Work out the finished part from the listing and answer in its coordinate system (mm). A direction names the side the tool comes from. Give positions to 0.01 mm unless a question says otherwise; leave off trailing zeros. Order: outer loops, then holes, each group sorted by start corner. A loop starts at its lowest first (then second) coordinate and runs counter-clockwise, first axis right, second up. Notation, with made-up numbers: (28.25, -23.5) - (33.25, -23.5) arc R28 ccw to (33.25, 14.5) - close; hole circle Ø6 at (68.25, 11.25). An arc over 180 degrees is marked (long way). Write each question's results on one line, items separated by ' | '.
from build123d import *
from build123d.topology import SkipClean

# Parameters (mm, degrees)
SKETCH1_W           = 18
SKETCH1_H           = 20
BOSS_EXTRUDE1_DEPTH = 18
SKETCH6_R           = 7.25
BOSS_EXTRUDE4_DEPTH = 12
FILLET1_R           = 2
SKETCH2_R           = 6.575
SKETCH2_R_2         = 5.625
BOSS_EXTRUDE5_DEPTH = 10
BOSS_EXTRUDE6_START = 10
SKETCH3_R           = 6.575
SKETCH3_R_2         = 5.625
BOSS_EXTRUDE6_DEPTH = 10
SKETCH7_R           = 5.625
CUT_EXTRUDE2_DEPTH  = 41
SKETCH8_W           = 18
SKETCH8_H           = 20
BOSS_EXTRUDE7_DEPTH = 3


with BuildPart() as part:
    # Sketch1 → Boss-Extrude1 (new body)
    with BuildSketch(Plane(origin=(0, 0, 0), x_dir=(1, 0, 0), z_dir=(0, 1, 0))):
        Rectangle(SKETCH1_W, SKETCH1_H)
    extrude(amount=BOSS_EXTRUDE1_DEPTH)

    # Sketch6 → Boss-Extrude4 (add)
    with BuildSketch(Plane(origin=(0, 18, 0), x_dir=(1, 0, 0), z_dir=(0, 1, 0))):
        with Locations(Location((0, 0, 0), (0, 0, 270))):
            Circle(SKETCH6_R)
    extrude(amount=BOSS_EXTRUDE4_DEPTH)

    # Fillet1
    fillet1_edges = [part.edges().sort_by_distance(p)[0] for p in [
        (0, 18, -7.25),
        (0, 30, -7.25),
    ]]
    fillet(fillet1_edges, radius=FILLET1_R)

    # Sketch2 → Boss-Extrude5 (add)
    with BuildSketch(Plane.XY.offset(10)):
        with Locations(Location((0, 9, 0), (0, 0, 180))):
            Circle(SKETCH2_R)
        with Locations((0, 9)):
            Circle(SKETCH2_R_2, mode=Mode.SUBTRACT)
    extrude(amount=BOSS_EXTRUDE5_DEPTH)

    # Sketch3 → Boss-Extrude6 (add)
    with BuildSketch(Plane(origin=(0, 0, -10), x_dir=(-1, 0, 0), z_dir=(0, 0, -1)).offset(BOSS_EXTRUDE6_START)):
        with Locations((0, 9)):
            Circle(SKETCH3_R)
        with Locations(Location((0, 9, 0), (0, 0, 180))):
            Circle(SKETCH3_R_2, mode=Mode.SUBTRACT)
    extrude(amount=-BOSS_EXTRUDE6_DEPTH)

    # Sketch7 → Cut-Extrude2 (cut)
    with SkipClean():  # the faces are left unmerged after this step: merging them gives an invalid solid
        with BuildSketch(Plane(origin=(0, 0, -10), x_dir=(-1, 0, 0), z_dir=(0, 0, -1))):
            with Locations((0, 9)):
                Circle(SKETCH7_R)
        extrude(amount=-CUT_EXTRUDE2_DEPTH, mode=Mode.SUBTRACT)

    # Sketch8 → Boss-Extrude7 (add)
    with SkipClean():  # the faces are left unmerged after this step: merging them gives an invalid solid
        with BuildSketch(Plane.XZ):
            Rectangle(SKETCH8_W, SKETCH8_H)
        extrude(amount=BOSS_EXTRUDE7_DEPTH)


solid = part.part
1. A cutting plane is placed at B-B, the plane y = 14. Write down the section's boundary in (x, z), then the cut area to 3 significant figures.
Answer list:
outline: (-9, -10) - (-4.27, -10) - (-4.27, -20) - (-2.58, -20) - (-2.58, 20) - (-4.27, 20) - (-4.27, 10) - (-9, 10) - close; (2.58, -20) - (4.27, -20) - (4.27, -10) - (9, -10) - (9, 10) - (4.27, 10) - (4.27, 20) - (2.58, 20) - close | area: 325 mm^2
2. A cutting plane is placed at A-A, the plane x = 0. Write down the section's boundary in (y, z) (3 decimals).
Answer list:
outline: (-3, -10) - (2.425, -10) - (2.425, -20) - (3.375, -20) - (3.375, 20) - (2.425, 20) - (2.425, 10) - (-3, 10) - close; (14.625, -20) - (15.575, -20) - (15.575, -10) - (18, -10) - (18, -9.25) arc R2 cw to (20, -7.25) - (28, -7.25) arc R2 ccw to (30, -5.25) - (30, 5.25) arc R2 ccw to (28, 7.25) - (20, 7.25) arc R2 cw to (18, 9.25) - (18, 10) - (15.575, 10) - (15.575, 20) - (14.625, 20) - close
3. Straight lines are drawn through the part: line 1 (X direction, y = 9, z = -5.5) (3 decimals); line 2 (Y direction, x = 0, z = 4.5) (3 decimals); line 3 (Y direction, x = 0, z = -12.5) (3 decimals). For each, find the intervals that lie inside material, in ascending order. Write a range as [from, to].
Answer list:
line 1: [-9, -5.625], [5.625, 9] | line 2: [-3, 3.375], [14.625, 30] | line 3: [2.425, 3.375], [14.625, 15.575]
4. Given P1, Ø8, axis at x = -1.5, y = 23.5, coming from the +Z side; P2, Ø9, axis at x = 0, y = 9, coming from the -Z side; P3, Ø3, axis at x = 1.5, y = 26.5, coming from the -Z side, each flat-ended and moving along its own axis, determine where each tip first touches the part or whether it passes through.
Answer list:
P1: z = 7.27 | P2: through | P3: z = -7.25
5. A cutting plane is placed at C-C, the plane z = -15.5. Write down the section's boundary in (x, y) (3 decimals).
Answer list:
outline: circle Ø13.15 at (0, 9); hole circle Ø11.25 at (0, 9)
6. A tool of negligible diameter and unlimited length cuts with its end or side. For faces 1 (the face through (-4, 3, -10)), 2 (the face through (1.425, 15.419, 14.93)), 3 (the face through (-2.777, 23.932, 6.697)), 4 (the face through (-1.4, 18, -9.3)), from which of +Z, -Z, +X, -X, +Y, -Y can it reach the whole face along a straight path? Write none if from no direction.
Answer list:
face 1: -Z | face 2: +Z | face 3: +Y | face 4: -Z, +Y
